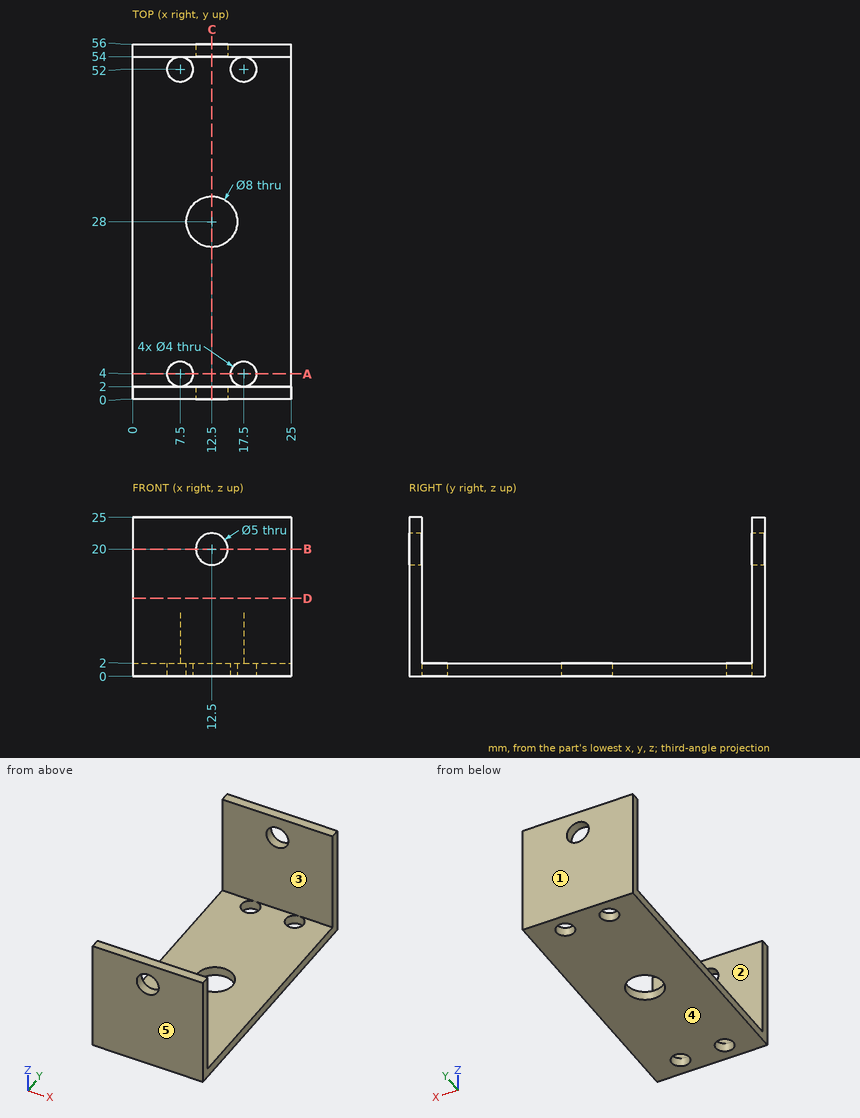
Source: three-view drawing plus pictorial views. Frame: mm from the lowest corner of the part. A direction names the side the tool comes from. Give positions to 0.01 mm unless a question says otherwise; leave off trailing zeros. Loops run counter-clockwise (first coordinate to the right, second up) from the corner with the lowest first, then second, coordinate; pieces in that order, holes last. Notation, with made-up numbers: (80.5, -29) -> (120.5, -29) arc R24 cw to (120.5, 7) -> close; hole circle Ø10 at (63.25, 65). An arc over 180 degrees is marked (long way). Put each result on its own line as item: value. Start each with the question number.
1) Draft query along Y for the marked faces 3, 4 and 5. Return one class per face: released by +Y, released by -Y, zero draft, split by the parting line, or undercut.
2) Contact query for flat-ended pins moving along their axis: P1, Ø3, axis at x = 7.5, y = 4, coming from the +Z side; P2, Ø5, axis at x = 3, y = 13, coming from the +Z side. Output: stop coordinate, or through.
3) Cut plane C-C (x = 12.5). Return loops of the section in (y, z), then the cut area to 3 significant figures.
4) Material intervals for probe 1 along X at (y, z) = (4, 1.5); probe 2 along Y at (x, z) = (5.5, 5); probe 3 along X at (y, z) = (0.9, 20), sorted ascending.
5) Reachability of the marked faces 1 and 2 from +Z, -Z, +X, -X, +Y, -Y: full face, straight path, thin tool, end or side. Return the list, or none.
6) Cut plane A-A (y = 4). Return loops of the section in (x, z), then the cut area to 3 significant figures.
7) Cut plane D-D (z = 12.25). Return loops of the section in (x, y).
8) Cut plane B-B (z = 20). Return loops of the section in (x, y).
Results are:
1. face 3: undercut
1. face 4: zero draft
1. face 5: released by -Y
2. P1: passes through
2. P2: stops at z = 2
3. outline: (0, 0) -> (24, 0) -> (24, 2) -> (2, 2) -> (2, 17.5) -> (0, 17.5) -> close; (0, 22.5) -> (2, 22.5) -> (2, 25) -> (0, 25) -> close; (32, 0) -> (56, 0) -> (56, 17.5) -> (54, 17.5) -> (54, 2) -> (32, 2) -> close; (54, 22.5) -> (56, 22.5) -> (56, 25) -> (54, 25) -> close
3. area: 168 mm2
4. probe 1: x = 0 to 5.5, 9.5 to 15.5, 19.5 to 25
4. probe 2: y = 0 to 2, 54 to 56
4. probe 3: x = 0 to 10, 15 to 25
5. face 1: +Z, -Z, +X, -X, +Y
5. face 2: +Z, +X, -X
6. outline: (0, 0) -> (5.5, 0) -> (5.5, 2) -> (0, 2) -> close; (9.5, 0) -> (15.5, 0) -> (15.5, 2) -> (9.5, 2) -> close; (19.5, 0) -> (25, 0) -> (25, 2) -> (19.5, 2) -> close
6. area: 34.0 mm2
7. outline: (0, 0) -> (25, 0) -> (25, 2) -> (0, 2) -> close; (0, 54) -> (25, 54) -> (25, 56) -> (0, 56) -> close
8. outline: (0, 0) -> (10, 0) -> (10, 2) -> (0, 2) -> close; (0, 54) -> (10, 54) -> (10, 56) -> (0, 56) -> close; (15, 0) -> (25, 0) -> (25, 2) -> (15, 2) -> close; (15, 54) -> (25, 54) -> (25, 56) -> (15, 56) -> close
